Check sheet for the modelled part. Datum: model origin and axes. Units: mm. Face numbers are marked on the shaded views. A direction names the side the tool comes from. Round coordinates to 2 decimals unless told otherwise and drop trailing zeros. Loops run counter-clockwise (first coordinate to the right, second up) from the corner with the lowest first, then second, coordinate; pieces in that order, holes last. Notation, with made-up numbers: (28, 78) -> (42, 78) arc R28 cw to (42, 103) -> close; hole circle Ø3 at (13.5, 5). An arc over 180 degrees is marked (long way). Use one line per item in the form item = value. Start each with the question number.
(1) Material ranges on probe 1 along Y at (x, z) = (-24, -19.05); probe 2 along Z at (x, y) = (-25.4, 4); probe 3 along Y at (x, z) = (-29, -27), recorded low to high. Write a range as [from, to].
(2) Go/stop test with flat-tipped pins: pin 1 (7 mm diameter, centred on x = -25.4, z = -31.75, fed in from -Y); pin 2 (3 mm diameter, centred on y = 17.5, z = -4, fed in from +X). Record where each tip stops, or that it passes through.
(3) Sectioned sample at D-D (x = -24.5). Record the cut outline in (y, z), and give its area (3 significant figures).
(4) Draft check along Y on the marked faces 1, 2 and 3. Enter one of: released by +Y, released by -Y, zero draft, split by the parting line, or undercut.
(5) Sectioned sample at C-C (y = 7). Record the cut outline in (x, z), and give its area (3 significant figures).
(6) Sectioned sample at B-B (z = -6.35). Record the cut outline in (x, y) (3 decimals), and give its area (3 significant figures).
(7) Set-up check for the marked faces 4 and 5: record each of +Z, -Z, +X, -X, +Y, -Y from which the full face is reachable in a straight line by a thin tool's end or side.
(8) Sectioned sample at A-A (y = 17.78). Record the cut outline in (x, z).
Autodesk Inventor part; units mm, degrees
ref_plane "YZ Plane" through (0, 0, 0) normal (1, 0, 0) x (0, 1, 0)
ref_plane "XZ Plane" through (0, 0, 0) normal (0, 1, 0) x (-1, 0, 0)
ref_plane "XY Plane" through (0, 0, 0) normal (0, 0, 1) x (1, 0, 0)
sketch "Sketch1" plane through (0, 0, 0) normal (0, 1, 0) x (-1, 0, 0)
  line L0 (0, 0) -> (38.1, 0)
  line L1 (38.1, 0) -> (38.1, -38.1)
  line L2 (38.1, -38.1) -> (0, -38.1)
  line L3 (0, -38.1) -> (0, 0)
  line L4 (0, -38.1) -> (0, -31.75)
  line L5 (0, -38.1) -> (6.35, -38.1) construction
  line L6 (0, -31.75) -> (25.4, -31.75)
  line L7 (25.4, -31.75) -> (25.4, -6.35)
  dimension "d0" = 38.1
  dimension "d1" = 38.1
  dimension "d2" = 6.35
  dimension "d3" = 90
  dimension "d4" = 25.4
  dimension "d5" = 90
  dimension "d6" = 25.4
extrude "Extrusion1" add sketch "Sketch1" along normal blind 56.896
hole "Hole1" at (-25.4, 0, -31.75) at (-25.4, 0, -6.35) direction (0, 1, 0) diameter 7.9375 depth 12.7
sketch "Sketch2" plane through (-38.1, 0, -38.1) normal (-1, 0, 0) x (0, 0, 1)
  line L0 (38.1, 0) -> (0, 0)
  line L1 (19.05, 0) -> (19.05, 17.78)
  line L2 (19.05, 0) -> (36.83, 0) construction
  line L3 (19.05, 17.78) -> (19.05, 27.432)
  line L4 (19.05, 17.78) -> (28.702, 17.78) construction
  line L5 (19.05, 27.432) -> (19.05, 32.512)
  line L6 (19.05, 32.512) -> (19.05, 42.164)
  circle A0 centre (19.05, 17.78) radius 9.652
  circle A1 centre (19.05, 42.164) radius 9.652
  ellipse E0 centre (19.05, 42.164) end of major axis (28.702, 42.164) minor radius 3.5267
  ellipse E1 centre (19.05, 17.78) end of major axis (28.702, 17.78) minor radius 3.6751
  line L7 (19.05, 42.164) -> (19.05, 56.896)
  dimension "d16" = 17.78
  dimension "d17" = 90
  dimension "d18" = 9.652
  dimension "d19" = 90
  dimension "d20" = 5.08
  dimension "d21" = 180
  dimension "d22" = 9.652
  dimension "d23" = 180
  dimension "d32" = 14.732
extrude "Extrusion2" cut sketch "Sketch2" against normal blind 31.75
extrude "Extrusion3" cut sketch "Sketch2" against normal blind 38.1 contours E1 L3 L1 | L1 L3 E1 | E0 L7 L6 | L6 L7 E0
sketch "Sketch3" plane through (0, 0, 0) normal (1, 0, 0) x (0, 0, -1)
  line L0 (38.1, 0) -> (38.1, 56.896)
  line L1 (0, 44.069) -> (38.1, 44.069)
  line L2 (38.1, 44.069) -> (38.1, 40.259)
  line L3 (38.1, 40.259) -> (0, 40.259)
  line L4 (0, 40.259) -> (0, 44.069)
  line L5 (0, 44.069) -> (38.1, 40.259) construction
  line L6 (38.1, 44.069) -> (0, 40.259) construction
  line L7 (0, 19.685) -> (38.1, 19.685)
  line L8 (38.1, 19.685) -> (38.1, 15.875)
  line L9 (38.1, 15.875) -> (0, 15.875)
  line L10 (0, 15.875) -> (0, 19.685)
  line L11 (0, 19.685) -> (38.1, 15.875) construction
  line L12 (38.1, 19.685) -> (0, 15.875) construction
  point P0 (0, 0)
  point P1 (19.05, 17.78)
  point P2 (19.05, 42.164)
  dimension "d28" = 3.81
  dimension "d29" = 3.81
extrude "Extrusion4" cut sketch "Sketch3" against normal blind 6.35
properties part number "Valve Holder"
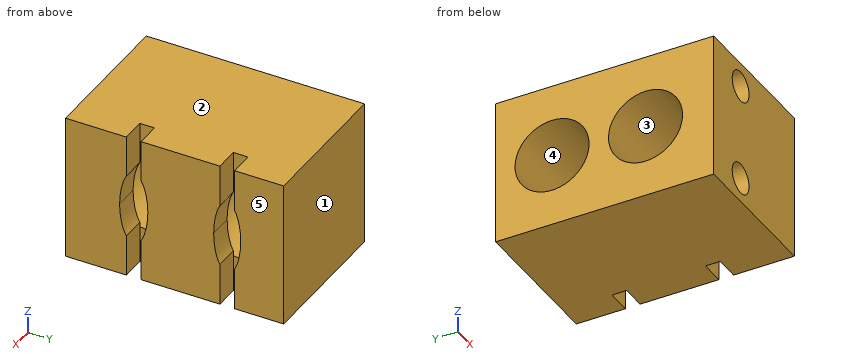
Checks:
q1.probe_1 = [0, 8.13], [27.43, 32.51], [51.82, 56.9]
q1.probe_2 = [-38.1, -35.72], [-27.78, -10.32], [-2.38, 0]
q1.probe_3 = [0, 12.31], [23.25, 36.69], [47.64, 56.9]
q2.pin_1 = 12.7
q2.pin_2 = -6.35
q3.outline = (0, -38.1) -> (56.9, -38.1) -> (56.9, 0) -> (0, 0) -> (0, -2.48) -> (12.7, -2.48) -> (12.7, -10.22) -> (0, -10.22) -> (0, -27.88) -> (12.7, -27.88) -> (12.7, -35.62) -> (0, -35.62) -> close; hole circle Ø19.3 at (17.78, -19.05); hole circle Ø19.3 at (42.16, -19.05)
q3.area = 1,390 mm2
q4.face_1 = released by +Y
q4.face_2 = zero draft
q4.face_3 = undercut
q5.outline = (-38.1, -38.1) -> (0, -38.1) -> (0, 0) -> (-38.1, 0) -> close; hole circle Ø7.94 at (-25.4, -31.75); hole circle Ø7.94 at (-25.4, -6.35)
q5.area = 1,350 mm2
q6.outline = (-38.1, 0) -> (-29.369, 0) -> (-29.369, 12.7) -> (-21.431, 12.7) -> (-21.431, 0) -> (0, 0) -> (0, 15.875) -> (-6.35, 15.875) -> (-6.35, 19.685) -> (0, 19.685) -> (0, 40.259) -> (-6.35, 40.259) -> (-6.35, 44.069) -> (0, 44.069) -> (0, 56.896) -> (-38.1, 56.896) -> close
q6.area = 2,020 mm2
q7.face_4 = -X
q7.face_5 = +Z, -Z, +X, +Y, -Y
q8.outline = (-38.1, -38.1) -> (-6.35, -38.1) -> (-6.35, -28.7) -> (-38.1, -28.7) -> close; (-38.1, -9.4) -> (-6.35, -9.4) -> (-6.35, 0) -> (-38.1, 0) -> close
